from build123d import *

# Parameters (mm, degrees)
BOSS_EXTRUDE1_DEPTH = 285.75
FILLET1_R           = 1.016


with BuildPart() as part:
    # Sketch1 → Boss-Extrude1 (new body)
    with BuildSketch(Plane.XY):
        with BuildLine():
            Line((0, 0), (0, 22.225))
            Line((0, 22.225), (1.3462, 22.225))
            Line((1.3462, 22.225), (1.3462, 11.684))
            Line((1.3462, 11.684), (9.2837, 11.684))
            Line((9.2837, 11.684), (9.2837, 12.7))
            Line((9.2837, 12.7), (2.3622, 12.7))
            Line((2.3622, 12.7), (2.3622, 23.241))
            Line((2.3622, 23.241), (-1.016, 23.241))
            Line((-1.016, 23.241), (-1.016, 1.016))
            Line((-1.016, 1.016), (-2.063377597, 1.016))
            ThreePointArc((-2.063377597, 1.016), (-2.48529022, 6.527253883), (-4.39485769, 11.714303305))
            ThreePointArc((-4.39485769, 11.714303305), (-6.222056703, 16.926496827), (-6.386074797, 22.44725))
            Line((-6.386074797, 22.44725), (-8.112125, 22.44725))
            Line((-8.112125, 22.44725), (-8.112125, 27.524569046))
            Line((-8.112125, 27.524569046), (2.744277132, 27.162688975))
            Line((2.744277132, 27.162688975), (2.778125, 28.178125))
            Line((2.778125, 28.178125), (-9.128125, 28.575))
            Line((-9.128125, 28.575), (-9.128125, 21.43125))
            Line((-9.128125, 21.43125), (-7.501829835, 21.43125))
            ThreePointArc((-7.501829835, 21.43125), (-7.107934178, 16.178984322), (-5.290870799, 11.235328872))
            ThreePointArc((-5.290870799, 11.235328872), (-3.370198099, 5.780137709), (-3.175, 0))
            Line((-3.175, 0), (0, 0))
        make_face()
    extrude(amount=-BOSS_EXTRUDE1_DEPTH)

    # Fillet1
    fillet1_edges = [part.edges().sort_by_distance(p)[0] for p in [
        (-3.175, 0, -142.875),
        (-9.128125, 21.43125, -142.875),
        (-6.386074797, 22.44725, -142.875),
        (-1.016, 23.241, -142.875),
        (2.3622, 23.241, -142.875),
        (1.3462, 11.684, -142.875),
        (0, 0, -142.875),
    ]]
    fillet(fillet1_edges, radius=FILLET1_R)


solid = part.part
For this review, take the finished solid that the model builds, in its own axes (mm). A direction names the side the tool comes from. Round coordinates to 2 decimals unless told otherwise and drop trailing zeros. Order: outer loops, then holes, each group sorted by start corner. A loop starts at its lowest first (then second) coordinate and runs counter-clockwise, first axis right, second up. Notation, with made-up numbers: M 55,-21.5 L 75,-21.5 A21 ccw 75,1.5 Z; hole C 78.5,23 d1. An arc over 180 degrees is marked long. Use a Markdown table: item, result. Add a question column.
Item 1: Insertion check: pin 1 (4 mm diameter, centred on x = 0.5, z = -243, fed in from +Y); pin 2 (1.5 mm diameter, centred on y = 17, z = -53.5, fed in from +X); pin 3 (2 mm diameter, centred on x = 6, z = -183.5, fed in from -Y). Each pin has a flat end and moves straight along its axis. Give the tip position at first contact, or say it passes through.
Item 2: Mouldability with a two-part tool opening along Y and no side actions: class faces 1 (the flat face through (6, 11.684, -141)), 2 (the flat face through (-0.6, 17.5, -285.75)), 3 (the flat face through (-8.112, 25, -141)) as released by +Y, released by -Y, zero draft, split by the parting line, or undercut.
Item 3: Tool access review of faces 4 (the flat face through (-1.016, 12, -141)), 5 (the flat face through (0, 11, -141)), 6 (the flat face through (2.362, 17, -141)): name each direction out of +Z, -Z, +X, -X, +Y, -Y from which nothing blocks a thin tool from reaching the whole face with its end or side.
Item 4: Add section A-A, the plane y = 15.5. Give the boundary of the cut face in (x, z), then the cut area to 3 significant figures.
Item 5: To check wall thickness, follow line 1 along X through (y, z) = (21.25, -100.5); line 2 along X through (y, z) = (16, -233); line 3 along Y through (x, z) = (-8, -245.5). State the ranges of each line that lie inside material, in increasing order.
Geometry results:
| question | item | result |
|---|---|---|
| 1 | pin 1 | stops at y = 28.32 |
| 1 | pin 2 | stops at x = 2.36 |
| 1 | pin 3 | stops at y = 11.68 |
| 2 | face 1 | released by -Y |
| 2 | face 2 | zero draft |
| 2 | face 3 | undercut |
| 3 | face 4 | +Z, -Z |
| 3 | face 5 | +Z, -Z, -Y |
| 3 | face 6 | +Z, -Z, +X |
| 4 | outline | M -6.95,-285.75 L -5.9,-285.75 L -5.9,0 L -6.95,0 Z; M -1.02,-285.75 L 0,-285.75 L 0,0 L -1.02,0 Z; M 1.35,-285.75 L 2.36,-285.75 L 2.36,0 L 1.35,0 Z |
| 4 | area | 881 mm² |
| 5 | line 1 | x = -7.51 to -6.49, -1.02 to 0, 1.35 to 2.36 |
| 5 | line 2 | x = -7.07 to -6.02, -1.02 to 0, 1.35 to 2.36 |
| 5 | line 3 | y = 21.43 to 22.45, 27.52 to 28.54 |
